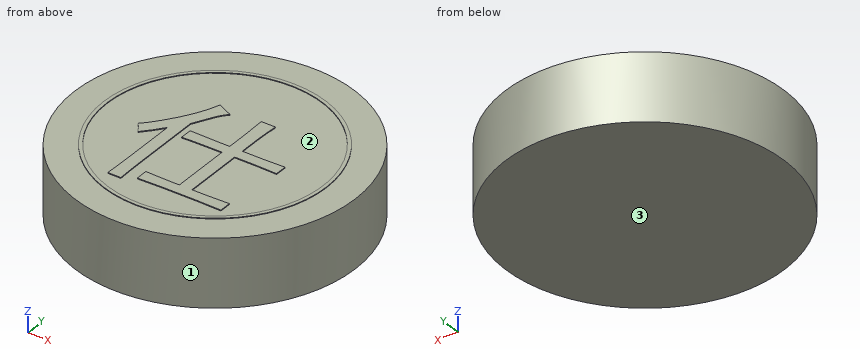
```python
from build123d import *

# Parameters (mm, degrees)
SKETCH_1_R               = 16.5
DIAMETER33_HEIGHT8_DEPTH = 8
CHARACTER_DEPTH          = 0.1
SKETCH_3_R               = 13.1
SKETCH_3_R_2             = 12.7
INK_RING_DEPTH           = 0.08


with BuildPart() as part:
    # 草图1 → Diameter33_Height8 (new body)
    with BuildSketch(Plane.XY):
        Circle(SKETCH_1_R)
    extrude(amount=-DIAMETER33_HEIGHT8_DEPTH)

    # 草图2 → Character_仕 (add)
    with BuildSketch(Plane.XY):
        with BuildLine():
            Line((1.385964912, 0.48245614), (1.385964912, 3.078947368))
            add(Edge.make_bspline(
                [(1.385964912, 3.078947368), (1.382856556, 3.540795331), (1.376713677, 4.453520939), (1.335934161, 5.365353156), (1.315789474, 5.815789474)],
                knots=[0, 0, 0, 0, 1.012019295, 2, 2, 2, 2], degree=3))
            Line((1.315789474, 5.815789474), (3, 5.815789474))
            add(Edge.make_bspline(
                [(3, 5.815789474), (2.977495606, 5.590667791), (2.932023515, 5.135789802), (2.894778649, 4.442009997), (2.862268379, 3.73162247), (2.860528273, 3.251395934), (2.859649123, 3.00877193)],
                knots=[0, 0, 0, 0, 0.965427312, 1.950730062, 2.964650972, 4, 4, 4, 4], degree=3))
            Line((2.859649123, 3.00877193), (2.859649123, 0.48245614))
            Line((2.859649123, 0.48245614), (5.385964912, 0.48245614))
            add(Edge.make_bspline(
                [(5.385964912, 0.48245614), (5.612960978, 0.48353494), (6.051396179, 0.485618604), (6.68734214, 0.499259504), (7.279297852, 0.517890937), (7.659345282, 0.541350279), (7.842105263, 0.552631579)],
                knots=[0, 0, 0, 0, 1.108393509, 2.14082447, 3.105946107, 4, 4, 4, 4], degree=3))
            Line((7.842105263, 0.552631579), (7.842105263, -0.850877193))
            add(Edge.make_bspline(
                [(7.842105263, -0.850877193), (7.659345282, -0.839595893), (7.279297852, -0.816136551), (6.68734214, -0.797505118), (6.051396179, -0.783864218), (5.612960978, -0.781780554), (5.385964912, -0.780701754)],
                knots=[0, 0, 0, 0, 0.894053893, 1.85917553, 2.891606491, 4, 4, 4, 4], degree=3))
            Line((5.385964912, -0.780701754), (2.859649123, -0.780701754))
            Line((2.859649123, -0.780701754), (2.859649123, -7.868421053))
            Line((2.859649123, -7.868421053), (4.403508772, -7.868421053))
            add(Edge.make_bspline(
                [(4.403508772, -7.868421053), (4.663425226, -7.867326084), (5.166829886, -7.865205357), (5.894610336, -7.851761208), (6.570572064, -7.832958173), (7.00263653, -7.809522024), (7.210526316, -7.798245614)],
                knots=[0, 0, 0, 0, 1.110647855, 2.151096232, 3.11039153, 4, 4, 4, 4], degree=3))
            Line((7.210526316, -7.798245614), (7.210526316, -9.201754386))
            add(Edge.make_bspline(
                [(7.210526316, -9.201754386), (7.010437031, -9.190419998), (6.583606619, -9.166241483), (5.90326924, -9.148137401), (5.144305253, -9.134624919), (4.612310457, -9.132626772), (4.333333333, -9.131578947)],
                knots=[0, 0, 0, 0, 0.835449614, 1.782180905, 2.836979614, 4, 4, 4, 4], degree=3))
            Line((4.333333333, -9.131578947), (0.263157895, -9.131578947))
            add(Edge.make_bspline(
                [(0.263157895, -9.131578947), (-0.015819229, -9.132626772), (-0.547814025, -9.134624919), (-1.306778012, -9.148137401), (-1.987115391, -9.166241483), (-2.413945803, -9.190419998), (-2.614035088, -9.201754386)],
                knots=[0, 0, 0, 0, 1.163020386, 2.217819095, 3.164550386, 4, 4, 4, 4], degree=3))
            Line((-2.614035088, -9.201754386), (-2.614035088, -7.798245614))
            add(Edge.make_bspline(
                [(-2.614035088, -7.798245614), (-2.407878143, -7.809517208), (-1.981010451, -7.832856124), (-1.318910587, -7.851574268), (-0.61279286, -7.865227274), (-0.127579839, -7.86733394), (0.122807018, -7.868421053)],
                knots=[0, 0, 0, 0, 0.904818853, 1.873514066, 2.902659025, 4, 4, 4, 4], degree=3))
            Line((0.122807018, -7.868421053), (1.385964912, -7.868421053))
            Line((1.385964912, -7.868421053), (1.385964912, -0.780701754))
            Line((1.385964912, -0.780701754), (-0.298245614, -0.780701754))
            add(Edge.make_bspline(
                [(-0.298245614, -0.780701754), (-0.452461393, -0.780188061), (-0.752239456, -0.7791895), (-1.189731892, -0.786231443), (-1.603011279, -0.790357704), (-1.992035716, -0.797879868), (-2.356713286, -0.809539056), (-2.697351984, -0.817728412), (-3.014316789, -0.834938878), (-3.217890625, -0.845701458), (-3.315789474, -0.850877193)],
                knots=[0, 0, 0, 0, 1.226022714, 2.383249742, 3.478491498, 4.511863319, 5.476544353, 6.379262498, 7.220585815, 8, 8, 8, 8], degree=3))
            Line((-3.315789474, -0.850877193), (-3.315789474, 0.552631579))
            add(Edge.make_bspline(
                [(-3.315789474, 0.552631579), (-3.21875707, 0.547453703), (-3.016916501, 0.536683017), (-2.703415706, 0.519544836), (-2.367110401, 0.511265445), (-2.010227251, 0.49975938), (-1.630736813, 0.492055864), (-1.229584063, 0.488016267), (-0.805954579, 0.480955843), (-0.51657237, 0.481948131), (-0.368421053, 0.48245614)],
                knots=[0, 0, 0, 0, 0.790917863, 1.645216496, 2.555317213, 3.528854326, 4.55156314, 5.644660669, 6.794166974, 8, 8, 8, 8], degree=3))
            Line((-0.368421053, 0.48245614), (1.385964912, 0.48245614))
        make_face()
        with BuildLine():
            add(Edge.make_bspline(
                [(-1.842105263, 5.114035088), (-1.933851435, 5.029026304), (-2.117541902, 4.858825164), (-2.365563333, 4.57167672), (-2.591993254, 4.259206087), (-2.763277727, 3.974023896), (-2.899956693, 3.72227062), (-3.016573333, 3.503293196), (-3.149738899, 3.257168631), (-3.294556387, 2.980814576), (-3.455706316, 2.678049907), (-3.630506142, 2.346123327), (-3.820034881, 1.98606085), (-3.950103328, 1.735288634), (-4.01754386, 1.605263158)],
                knots=[0, 0, 0, 0, 1.083759172, 2.169858686, 3.283228111, 4.425909641, 5.051182283, 5.766997595, 6.57693099, 7.477449721, 8.472081343, 9.550673888, 10.730023607, 12, 12, 12, 12], degree=3))
            Line((-4.01754386, 1.605263158), (-4.01754386, -6.464912281))
            add(Edge.make_bspline(
                [(-4.01754386, -6.464912281), (-4.018056133, -6.65204931), (-4.019052245, -7.015935362), (-4.012047973, -7.545266441), (-4.007901436, -8.042578811), (-4.000400634, -8.506973521), (-3.988771218, -8.938370958), (-3.98063319, -9.336170915), (-3.963429216, -9.700804491), (-3.952560119, -9.932966081), (-3.947368421, -10.043859649)],
                knots=[0, 0, 0, 0, 1.25452393, 2.439409025, 3.548794241, 4.588568869, 5.552973603, 6.441898353, 7.255762113, 8, 8, 8, 8], degree=3))
            Line((-3.947368421, -10.043859649), (-5.49122807, -10.043859649))
            add(Edge.make_bspline(
                [(-5.49122807, -10.043859649), (-5.48604403, -9.933832078), (-5.4752279, -9.704267368), (-5.458045854, -9.34570061), (-5.449866698, -8.958296312), (-5.43824574, -8.54249494), (-5.430714946, -8.098893278), (-5.426551478, -7.626704474), (-5.419547466, -7.12596442), (-5.420541736, -6.782003967), (-5.421052632, -6.605263158)],
                knots=[0, 0, 0, 0, 0.768562205, 1.603550436, 2.504569286, 3.472060047, 4.505901887, 5.600100741, 6.766834584, 8, 8, 8, 8], degree=3))
            Line((-5.421052632, -6.605263158), (-5.421052632, -0.219298246))
            add(Edge.make_bspline(
                [(-5.421052632, -0.219298246), (-5.477100123, -0.297465115), (-5.593729665, -0.460122996), (-5.780061764, -0.708596832), (-5.986068105, -0.970387502), (-6.216160665, -1.241667605), (-6.462173545, -1.53007964), (-6.726721569, -1.832063458), (-7.014400911, -2.14414193), (-7.213381091, -2.355918188), (-7.315789474, -2.464912281)],
                knots=[0, 0, 0, 0, 0.784966074, 1.633440328, 2.534521274, 3.503196048, 4.536232569, 5.628408604, 6.779421952, 8, 8, 8, 8], degree=3))
            add(Edge.make_bspline(
                [(-7.315789474, -2.464912281), (-7.376217454, -2.360289355), (-7.496986321, -2.151194296), (-7.698613752, -1.847907954), (-7.919509238, -1.554794995), (-8.078179419, -1.366518997), (-8.157894737, -1.271929825)],
                knots=[0, 0, 0, 0, 0.990939877, 1.980451519, 2.985386235, 4, 4, 4, 4], degree=3))
            add(Edge.make_bspline(
                [(-8.157894737, -1.271929825), (-8.078444276, -1.200683827), (-7.908680075, -1.048450351), (-7.650883543, -0.790792829), (-7.380450508, -0.484210357), (-7.085685528, -0.139123391), (-6.774453616, 0.251552056), (-6.444928694, 0.686800589), (-6.093822829, 1.163741111), (-5.733795482, 1.678782143), (-5.373823069, 2.211324676), (-5.038729415, 2.753088359), (-4.729340369, 3.291388528), (-4.443634689, 3.826106433), (-4.193529603, 4.362171988), (-3.965829486, 4.893831939), (-3.764036827, 5.42296806), (-3.651942432, 5.779680656), (-3.596491228, 5.956140351)],
                knots=[0, 0, 0, 0, 0.593635041, 1.268437926, 2.026139621, 2.86729733, 3.793145817, 4.804357063, 5.904290477, 7.087660503, 8.300109294, 9.479773153, 10.630579527, 11.753876596, 12.851315059, 13.920229824, 14.971172829, 16, 16, 16, 16], degree=3))
            add(Edge.make_bspline(
                [(-3.596491228, 5.956140351), (-3.455102142, 5.876001082), (-3.172790986, 5.715987251), (-2.737023645, 5.499372043), (-2.295481279, 5.293961951), (-1.99346903, 5.174105332), (-1.842105263, 5.114035088)],
                knots=[0, 0, 0, 0, 1.001016569, 1.998726716, 2.996993449, 4, 4, 4, 4], degree=3))
        make_face()
    extrude(amount=CHARACTER_DEPTH)

    # 草图3 → Ink_ring (add)
    with BuildSketch(Plane.XY):
        with Locations(Location((0, 0, 0), (0, 0, 180))):
            Circle(SKETCH_3_R)
        with Locations(Location((0, 0, 0), (0, 0, 180))):
            Circle(SKETCH_3_R_2, mode=Mode.SUBTRACT)
    extrude(amount=INK_RING_DEPTH)


solid = part.part
```
Build history of the part. All positions in model axes, mm. Face numbers are marked on the shaded views. Round coordinates to 2 decimals unless told otherwise and drop trailing zeros. Write each loop counter-clockwise with the first axis right and the second up, starting at its lowest first coordinate (ties: lowest second). Pieces come first, ordered by that corner, then holes.
1) Band-saw the part on B-B, the plane z = -6.75. List the corners of the cut face in (x, y), and give its area (3 significant figures).
2) Drill centre lines: probe 1 along Z at (x, y) = (10, -1.5); probe 2 along Y at (x, z) = (0, -6.25); probe 3 along X at (y, z) = (14.5, -4.25). Where is each one in solid material? Low to high.
3) Band-saw the part on D-D, the plane y = -4.5. List the corners of the cut face in (x, z).
4) Band-saw the part on A-A, the plane y = 9. List the corners of the cut face in (x, z).
5) Band-saw the part on C-C, the plane x = -11. List the corners of the cut face in (y, z).
6) Mould opens along X. For the marked faces 1, 2 and 3 say: +X half, -X half, draft (parallel to the pull), parting line (faces both ways), or undercut.
7) Pin check, flat tips, straight feed: pin 1 (2 mm diameter, centred on y = -5.5, z = -5.5, fed in from +X); pin 2 (1 mm diameter, centred on y = -10.5, z = -3, fed in from +X); pin 3 (1 mm diameter, centred on x = 9, z = -1, fed in from +Y). Stop position of each tip, or through.
Ans:
1. outline: circle Ø33 at (0, 0)
1. area: 855 mm2
2. probe 1: z = -8 to 0
2. probe 2: y = -16.5 to 16.5
2. probe 3: x = -7.87 to 7.87
3. outline: (-15.87, -8) - (15.87, -8) - (15.87, 0) - (12.3, 0) - (12.3, 0.08) - (11.88, 0.08) - (11.88, 0) - (2.86, 0) - (2.86, 0.1) - (1.39, 0.1) - (1.39, 0) - (-4.02, 0) - (-4.02, 0.1) - (-5.42, 0.1) - (-5.42, 0) - (-11.88, 0) - (-11.88, 0.08) - (-12.3, 0.08) - (-12.3, 0) - (-15.87, 0) - close
4. outline: (-13.83, -8) - (13.83, -8) - (13.83, 0) - (9.52, 0) - (9.52, 0.08) - (8.96, 0.08) - (8.96, 0) - (-8.96, 0) - (-8.96, 0.08) - (-9.52, 0.08) - (-9.52, 0) - (-13.83, 0) - close
5. outline: (-12.3, -8) - (12.3, -8) - (12.3, 0) - (7.11, 0) - (7.11, 0.08) - (6.35, 0.08) - (6.35, 0) - (-6.35, 0) - (-6.35, 0.08) - (-7.11, 0.08) - (-7.11, 0) - (-12.3, 0) - close
6. face 1: parting line
6. face 2: undercut
6. face 3: draft
7. pin 1: stops at x = 15.87
7. pin 2: stops at x = 13.12
7. pin 3: stops at y = 14.14
